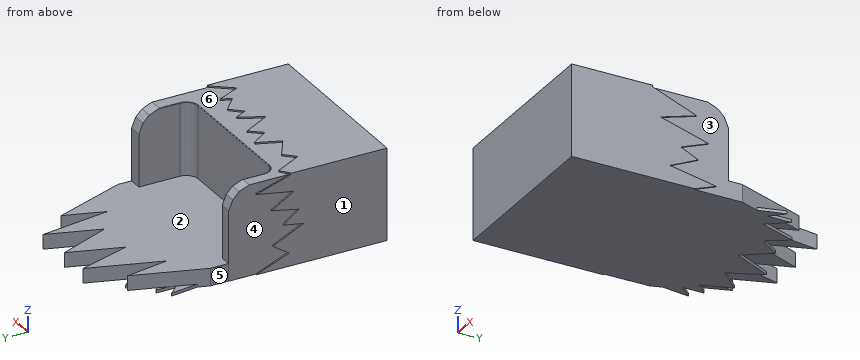
from build123d import *

# Parameters (mm, degrees)
F1_DEPTH  = 762
F3_DEPTH  = 127
F6_DEPTH  = 762.001
F8_DEPTH  = 25.4
F10_SIZE  = 127
F11_SIZE  = 50.8
F12_R     = 101.6
F13_R     = 5.08
F15_DEPTH = 12.7
F17_DEPTH = 12.7
F19_DEPTH = 12.7


with BuildPart() as f1:
    # F0 (on Top) → F1 (new body)
    with BuildSketch(Plane.XY):
        Polygon((-3498.5116661556, -1699.4458940506), (-3498.5116661556, -2613.8458940506), (-1974.5116661556, -2613.8458940506), (-1974.5116661556, -1699.4458940506), (-1974.5116661556, -1240.8709526062), (-2088.5074138641, -1240.8709526062), (-2088.5074138641, -1699.4458940506), (-3396.6603279114, -1705.0362136841), (-3396.6603279114, -1240.8709526062), (-3498.5116661556, -1240.8709526062), align=None)
    extrude(amount=F1_DEPTH)


with BuildPart() as f3:
    # F2 (on face) → F3 (new body)
    with BuildSketch(Plane(origin=(0, 0, 0), x_dir=(1, 0, 0), z_dir=(0, 0, -1))):
        Polygon((-1974.5116661556, 230.5383682251), (-1974.5116661556, 1240.8709526062), (-2088.5074138641, 1240.8709526062), (-2088.5074138641, 1699.4458940506), (-3396.6603279114, 1705.0362136841), (-3396.6603279114, 1240.8709526062), (-3496.481180191, 1240.8709526062), (-3496.481180191, 230.5383682251), align=None)
    extrude(amount=-F3_DEPTH)


with BuildPart() as f1_1:
    add(f1.part)

    # F4: union F3
    add(f3.part)

    # F5 (on face) → F6 (cut, through all)
    with BuildSketch(Plane(origin=(0, 0, 0), x_dir=(1, 0, 0), z_dir=(0, 0, -1))):
        Polygon((-2316.2273000234, 841.8166545124), (-2401.6864299774, 230.5383682251), (-1974.5116661556, 230.5383682251), (-1974.5116661556, 1119.2854642868), (-2203.1452655792, 498.7692832947), align=None)
        Polygon((-2735.4964231733, 230.5383682251), (-2401.6864299774, 230.5383682251), (-2551.6629219055, 685.5093240738), align=None)
        Polygon((-3496.481180191, 230.5383682251), (-3027.2831916809, 230.5383682251), (-3231.0576103647, 848.7115289264), (-3295.5253124237, 471.2162911892), (-3496.481180191, 1080.8390531707), align=None)
        Polygon((-3027.2831916809, 230.5383682251), (-2735.4964231733, 230.5383682251), (-2885.4729151014, 685.5093240738), align=None)
    extrude(amount=-F6_DEPTH, mode=Mode.SUBTRACT)


with BuildPart() as f8:
    # F7 (on face) → F8 (new body)
    with BuildSketch(Plane(origin=(0, 0, 0), x_dir=(1, 0, 0), z_dir=(0, 0, -1))):
        Polygon((-2905.2052497864, 390.9881711006), (-2834.7314291205, 531.5791842156), (-2885.4729151014, 685.5093240738), (-2947.5236220314, 486.4315835605), align=None)
        Polygon((-3214.7448062897, 498.7692832947), (-3141.0519449936, 575.6689801958), (-3231.0576103647, 848.7115289264), (-3264.8577193286, 650.7925747624), align=None)
        Polygon((-3413.8304513223, 830.1085511328), (-3465.3007291058, 986.2495648338), (-3496.481180191, 743.8611740208), align=None)
        Polygon((-3368.3185893378, 692.043077782), (-3396.0032463074, 776.02767218), (-3396.0032463074, 663.1536888734), align=None)
        Polygon((-2571.4828968048, 498.7692832947), (-2515.293202418, 575.1775925706), (-2551.6629219055, 685.5093240738), (-2606.951311997, 548.6756592969), align=None)
        Polygon((-2325.264623755, 490.6849679948), (-2259.4031983079, 669.4341994996), (-2316.2273000234, 841.8166545124), (-2357.9744639194, 543.2045013416), align=None)
        Polygon((-2078.1543254852, 837.9972051805), (-2128.849476835, 700.4095461938), (-2078.1543254852, 632.8159570694), align=None)
        Polygon((-2033.3765220407, 959.5250631011), (-2077.148481374, 840.727086301), (-1974.5116661556, 729.5470237732), align=None)
        Polygon((-2259.4031983079, 669.4341994996), (-2208.7411880493, 806.931912899), (-2128.849476835, 700.4095461938), (-2078.1543254852, 837.9972051805), (-2078.1543254852, 841.8166545124), (-2077.148481374, 840.727086301), (-2033.3765220407, 959.5250631011), (-1974.5116661556, 1119.2854642868), (-1974.5116661556, 2613.8458940506), (-3498.5116661556, 2613.8458940506), (-3498.5116661556, 1240.8709526062), (-3496.481180191, 1240.8709526062), (-3496.481180191, 1080.8390531707), (-3465.3007291058, 986.2495648338), (-3413.8304513223, 830.1085511328), (-3396.0032463074, 848.7115289264), (-3396.0032463074, 776.02767218), (-3368.3185893378, 692.043077782), (-3301.4554118653, 761.8158887578), (-3264.8577193286, 650.7925747624), (-3231.0576103647, 848.7115289264), (-3141.0519449936, 575.6689801958), (-3035.7921123505, 685.5093240738), (-2947.5236220314, 486.4315835605), (-2885.4729151014, 685.5093240738), (-2834.7314291205, 531.5791842156), (-2735.4964231733, 729.5470237732), (-2606.951311997, 548.6756592969), (-2551.6629219055, 685.5093240738), (-2515.293202418, 575.1775925706), (-2440.8960342407, 676.3449311256), (-2357.9744639194, 543.2045013416), (-2316.2273000234, 841.8166545124), align=None)
    extrude(amount=F8_DEPTH)

    # F9: union F1
    add(f1_1.part)

    # F10
    f10_edges = [f8.edges().sort_by_distance(p)[0] for p in [
        (-3447.585997, -1240.870953, 762),
        (-2031.50954, -1240.870953, 762),
    ]]
    chamfer(f10_edges, length=F10_SIZE)

    # F11
    f11_edges = [f8.edges().sort_by_distance(p)[0] for p in [
        (-2031.50954, -1240.870953, 635),
        (-2031.50954, -1367.870953, 762),
        (-3447.585997, -1240.870953, 635),
        (-3447.585997, -1367.870953, 762),
    ]]
    chamfer(f11_edges, length=F11_SIZE)

    # F12
    f12_edges = [f8.edges().sort_by_distance(p)[0] for p in [
        (-3396.660328, -1705.036214, 444.5),
        (-2088.507414, -1699.445894, 444.5),
    ]]
    fillet(f12_edges, radius=F12_R)

    # F13
    f13_edges = [f8.edges().sort_by_distance(p)[0] for p in [
        (-2742.149693, -1702.239198, 762),
    ]]
    fillet(f13_edges, radius=F13_R)

    # F14 (on face) → F15 (join)
    with BuildSketch(Plane.YZ.offset(-1974.5116661556)):
        Polygon((-1524.0049362183, 610.3619337082), (-1908.9328050613, 762), (-2613.8458940506, 762), (-2613.8458940506, -25.4), (-1540.454864502, -25.4), (-1352.9258966446, 44.4850027561), (-1757.5936317444, 120.1545894146), (-1510.8450651169, 232.0139855146), (-1662.1842384338, 304.3935894966), (-1418.6709526062, 396.5130746365), (-1839.8432731628, 518.242418766), align=None)
    extrude(amount=F15_DEPTH)

    # F16 (on face) → F17 (join)
    with BuildSketch(Plane(origin=(-3498.5116661556, 0, 0), x_dir=(0, -1, 0), z_dir=(-1, 0, 0))):
        Polygon((1758.8893175125, 87.9818573594), (1473.0749130249, -25.4), (2613.8458940506, -25.4), (2613.8458940506, 762), (1772.6634740829, 762), (1473.0749130249, 669.9413061142), (1803.6553859711, 611.4010214806), (1607.3732376099, 494.320422411), (1844.9779748917, 446.1107254028), (1710.6796503067, 342.8043425083), (1889.7440433502, 311.8124306202), (1617.7039146423, 184.4011843204), align=None)
    extrude(amount=F17_DEPTH)

    # F18 (on face) → F19 (join)
    with BuildSketch(Plane.XY.offset(762)):
        Polygon((-3426.700592041, -1715.4284715652), (-3498.5116661556, -1772.6634740829), (-3511.2116661556, -1772.6634740829), (-3511.2116661556, -2613.8458940506), (-1961.8116661556, -2613.8458940506), (-1961.8116661556, -1908.9328050613), (-1974.5116661556, -1908.9328050613), (-2110.2046966553, -2084.5901966095), (-2202.495098114, -1886.4371776581), (-2242.4262828624, -1971.1439244185), (-2373.5039234161, -1853.8640737534), (-2465.7943248749, -1957.012295723), (-2517.3683166504, -1853.8640737534), (-2620.51653862, -2052.0172119141), (-2753.523349762, -1815.8621788025), (-2837.6703262329, -1921.7246770859), (-2943.5329437256, -1772.6634740829), (-3024.965763092, -1976.0131835938), (-3209.5465660095, -1862.0073795319), (-3299.1225719452, -1954.2977809906), align=None)
    extrude(amount=F19_DEPTH)


solid = f8.part
For this review, take the finished solid that the model builds, in its own axes (mm). Face numbers are marked on the shaded views. A direction names the side the tool comes from. Round coordinates to 2 decimals unless told otherwise and drop trailing zeros. Order: outer loops, then holes, each group sorted by start corner. A loop starts at its lowest first (then second) coordinate and runs counter-clockwise, first axis right, second up. Notation, with made-up numbers: (-7.5, 27.25) -> (-3.5, 27.25) arc R20 ccw to (-3.5, 53.25) -> close; hole circle Ø7 at (-21, -22.75). An arc over 180 degrees is marked (long way). Put each result on its own line as item: value.
Q1. Add section A-A on y = -931. Write out the cut boundary in (x, z), plus the area to 3 significant figures.
Check result:
outline: (-3472.41, -25.4) -> (-2026.08, -25.4) -> (-2026.08, 0) -> (-2043.89, 0) -> (-2043.89, 127) -> (-3447.09, 127) -> (-3447.09, 0) -> (-3472.41, 0) -> close
area: 215,000 mm2
Q2. Machinability: for the marked faces 4, 5 and 6, which of the approach directions +Z, -Z, +X, -X, +Y, -Y give a long, thin tool a straight path to every point of the face, cutting with its end or side? Answer none if there is none.
Check result:
face 4: -X, +Y
face 5: +Z, -Z, -X, +Y
face 6: +Z, +Y
Q3. Mouldability with a two-part tool opening along Z and no side actions: class the marked faces 1, 2 and 3 as pulls with the +Z half, pulls with the -Z half, needs draft (parallel to the pull), parting line crosses it, or undercut.
Check result:
face 1: needs draft
face 2: pulls with the +Z half
face 3: undercut
Q4. For probe 1 along X at (y, z) = (-1385.5, 401.5); probe 2 along Z at (x, y) = (-3264, -1308.5); probe 3 along Y at (x, z) = (-2288, 466), list the stretches that pass through material, from the lowest coordinate up. Write a range as [from, to].
Check result:
probe 1: [-3498.51, -3396.66], [-2088.51, -1974.51]
probe 2: [-25.4, 127]
probe 3: [-2613.85, -1700.3]
Q5. Insertion check: pin 1 Ø10 at (x, y) = (-2228.5, -949.5) entering from +Z; pin 2 Ø1 at (y, z) = (-1399.5, 579.5) entering from +X; pin 3 Ø12.5 at (y, z) = (-794.5, -16) entering from -X. Each pin has a flat end and moves straight along its axis. Give the tip position at first contact, or say it passes through.
Check result:
pin 1: z = 127
pin 2: x = -1974.51
pin 3: x = -3490.77
